```python
from build123d import *


# Not quite as in the source:
# - a fillet or chamfer that OpenCascade refuses, or shapes differently, is made with other operations: its cross-section is extruded or revolved along the edge and cut away or added


with BuildPart() as f1:
    # F0 (on Front) → F1 (revolve)
    with BuildSketch(Plane.XZ):
        with BuildLine():
            Line((0, 38.5912625485), (0, 0))
            Line((0, 0), (19.7524651885, 0))
            Line((19.7524651885, 0), (19.7524651885, 3.1980082858))
            Line((19.7524651885, 3.1980082858), (14.1919255257, 5.8136251755))
            Line((14.1919255257, 5.8136251755), (8.4569835516, 26.5488596043))
            ThreePointArc((8.4569835516, 26.5488596043), (5.8902046524, 30.3760769017), (6.9375761897, 34.8637220549))
            Line((6.9375761897, 34.8637220549), (8.4767341614, 36.9339473546))
            Line((8.4767341614, 36.9339473546), (6.2475829585, 38.5912625485))
            ThreePointArc((6.2475829585, 38.5912625485), (7.9366897799, 47.9479775999), (0, 53.183448328))
            Line((0, 53.183448328), (0, 38.5912625485))
        make_face()
    revolve(axis=Axis((0, 0, 19.2956312742), (0, 0, 1)))

    # F2: fillet of radius 19.7282149364 on 1 edges, made by hand

    # F2_s1 → F2_t2 (revolve)
    with BuildSketch(Plane.XZ):
        with BuildLine():
            ThreePointArc((19.7524651885, 3.1980082858), (14.8303095618, 8.0151476836), (11.8639351327, 14.2306984022))
            Line((11.8639351327, 14.2306984022), (11.4836480923, 14.1255187807))
            Line((11.4836480923, 14.1255187807), (13.8116384853, 5.708445554))
            Line((13.8116384853, 5.708445554), (14.0239794459, 5.4565886226))
            ThreePointArc((14.0239794459, 5.4565886226), (16.8042492773, 4.1487801778), (19.5299487493, 2.872174862))
            Line((19.5299487493, 2.872174862), (19.7524651885, 3.1980082858))
        make_face()
    revolve(axis=Axis((0, 0, 5.8136251755), (0, 0, 1)))


solid = f1.part
```
Verification items for the finished model (mm, model axes). Coordinates: 2 decimals unless noted, no trailing zeros. Write each loop counter-clockwise with the first axis right and the second up, starting at its lowest first coordinate (ties: lowest second). Pieces come first, ordered by that corner, then holes. Notation, with made-up numbers: M 69.25,42 L 79.25,42 A28 cw 79.25,80 Z; hole C -20.75,32 d10. An arc over 180 degrees is marked long. Answer as a JSON object with one key per item and string values. Group by question number.
(1) Cross-section at C-C, the plane z = 28. Record the cut outline in (x, y).
(2) Cross-section at D-D, the plane z = 17.5. Record the cut outline in (x, y).
(3) Material ranges on line 1 (Z direction, x = 0.5, y = 7.5); line 2 (Z direction, x = -17, y = 5); line 3 (Y direction, x = -3, z = 20), recorded low to high.
(4) Cross-section at A-A, the plane y = 0. Record the cut outline in (x, z), and give its area (3 significant figures).
(5) Release check for a two-part mould opening along Z. For faces 1 (the face through (5.9, -2.4, 38.5)), 2 (the face through (0, 0, 0)), 3 (the face through (-4.282, -19.283, 1.621)) record: +Z half, -Z half, draft (parallel to the pull), parting line (faces both ways), or undercut.
(6) Gauge pin test, flat ends, axial feed: pin 1 (10 mm diameter, centred on y = 3.5, z = 45.5, fed in from +X); pin 2 (6 mm diameter, centred on y = -12, z = 13, fed in from -X); pin 3 (5 mm diameter, centred on x = 1, z = 43.5, fed in from +Y). Record the tip position at first contact, or that the pin passes through.
Reply:
{
 "1": {"outline": "C 0,0 d13.83"},
 "2": {"outline": "C 0,0 d21.92"},
 "3": {"line 1": "0 to 27.3, 35.64 to 37.65, 40.3 to 48.8", "line 2": "0 to 4.79", "line 3": "-9.82 to 9.82"},
 "4": {"outline": "M -19.75,0 L 19.75,0 L 19.75,3.2 A19.73 cw 11.86,14.23 L 8.46,26.55 A5.78 cw 6.94,34.86 L 8.48,36.93 L 6.25,38.59 A8.63 ccw long -6.25,38.59 L -8.48,36.93 L -6.94,34.86 A5.78 cw -8.46,26.55 L -11.86,14.23 A19.73 cw -19.75,3.2 Z", "area": "1,080 mm²"},
 "5": {"face 1": "undercut", "face 2": "-Z half", "face 3": "draft"},
 "6": {"pin 1": "x = 8.63", "pin 2": "x = -8.75", "pin 3": "y = 8.63"}
}
